Here's how the part is built. I have some questions about the finished solid (model axes, mm). A direction names the side the tool comes from. Round coordinates to 2 decimals unless told otherwise and drop trailing zeros. Loops run counter-clockwise (first coordinate to the right, second up) from the corner with the lowest first, then second, coordinate; pieces in that order, holes last. Notation, with made-up numbers: (69, 70.25) -> (78, 70.25) arc R27 ccw to (78, 92.25) -> close; hole circle Ø1 at (88.25, 89). An arc over 180 degrees is marked (long way). Use CSV: the item, a comma, the result in double quotes. Start each with the question number.
from build123d import *

# Parameters (mm, degrees)
BOSS_EXTRUDE1_DEPTH = 63.5


with BuildPart() as part:
    # Sketch1 → Boss-Extrude1 (new, symmetric)
    with BuildSketch(Plane(origin=(0, 0, 0), x_dir=(0, 0, -1), z_dir=(1, 0, 0))):
        Polygon((0, 0), (250, 0), (250, -12.7), (0, -12.7), (-12.7, -12.7), (-12.7, 114.3), (0, 114.3), align=None)
    extrude(amount=BOSS_EXTRUDE1_DEPTH, both=True)


solid = part.part
Q1. For faces 1 (the flat face through (1, 0, -123)), 2 (the flat face through (1, 114.3, 6)), which set-ups out of +Z, -Z, +X, -X, +Y, -Y let a thin tool reach every point of the face, with its end or its side?
Q2. I need wall thicknesses on line 1 along Z through (x, y) = (27, 85.5); line 2 along Y through (x, z) = (-14, -73.5). Which ranges of each line are inside material? Lowest first, please.
Q3. I want a section at C-C, the plane z = -220. List the corners of the cut face in (x, y) for me, then the cut area to 3 significant figures.
Q4. I want a section at A-A, the plane x = 13.5. List the corners of the cut face in (y, z) for me, then the cut area to 3 significant figures.
Q5. I want a section at B-B, the plane y = 60.5. List the corners of the cut face in (x, z) for me.
Q6. Will this pin go through, and if not, where does the flat tip stop? pin 1 Ø1.5 at (x, y) = (-20, 4.5) entering from -Z.
Values found:
1,face 1,"-Z, +X, -X, +Y"
1,face 2,"+Z, -Z, +X, -X, +Y"
2,line 1,"0 to 12.7"
2,line 2,"-12.7 to 0"
3,outline,"(-63.5, -12.7) -> (63.5, -12.7) -> (63.5, 0) -> (-63.5, 0) -> close"
3,area,"1,610 mm2"
4,outline,"(-12.7, -250) -> (0, -250) -> (0, 0) -> (114.3, 0) -> (114.3, 12.7) -> (-12.7, 12.7) -> close"
4,area,"4,790 mm2"
5,outline,"(-63.5, 0) -> (63.5, 0) -> (63.5, 12.7) -> (-63.5, 12.7) -> close"
6,pin 1,"z = 0"
